```python
from build123d import *

# Parameters (mm, degrees)
EXTRUDE_1_DEPTH     = 2
SKETCH_2_W          = 90
SKETCH_2_H          = 11
CUT_EXTRUDE_1_DEPTH = 2
SKETCH_4_W          = 10
SKETCH_4_H          = 11
SKETCH_4_R          = 1.65
EXTRUDE_3_DEPTH     = 2
FILLET_2_R          = 2


with BuildPart() as part:
    # 草图1 → 凸台-拉伸1 (new body)
    with BuildSketch(Plane.XY):
        Polygon((-33, -15), (-52.5, -15), (-52.5, 15), (-33, 15), (-33, 17), (-23, 17), (-23, 15), (23, 15), (23, 17), (33, 17), (33, 15), (52.5, 15), (52.5, -15), (33, -15), (33, -17), (23, -17), (23, -15), (-23, -15), (-23, -17), (-33, -17), align=None)
    extrude(amount=EXTRUDE_1_DEPTH)

    # 草图2 → 切除-拉伸1 (cut)
    with BuildSketch(Plane.XY.offset(2)):
        Rectangle(SKETCH_2_W, SKETCH_2_H)
    extrude(amount=-CUT_EXTRUDE_1_DEPTH, mode=Mode.SUBTRACT)

    # 草图4 → 凸台-拉伸3 (add)
    # profile 1 of 2: a face of its own
    with BuildSketch(Plane(origin=(0, 0, 0), x_dir=(-1, 0, 0), z_dir=(0, 0, -1))):
        with Locations((-22.5, 0)):
            Rectangle(SKETCH_4_W, SKETCH_4_H)
        with Locations((-22.5, 0)):
            Circle(SKETCH_4_R, mode=Mode.SUBTRACT)
    # profile 2 of 2: a face of its own
    with BuildSketch(Plane(origin=(0, 0, 0), x_dir=(-1, 0, 0), z_dir=(0, 0, -1))):
        with Locations((22.5, 0)):
            Rectangle(SKETCH_4_W, SKETCH_4_H)
        with Locations((22.5, 0)):
            Circle(SKETCH_4_R, mode=Mode.SUBTRACT)
    extrude(amount=-EXTRUDE_3_DEPTH)

    # 圆角2
    fillet_2_edges = [part.edges().sort_by_distance(p)[0] for p in [
        (-45, -5.5, 1),
        (-45, 5.5, 1),
        (45, 5.5, 1),
        (45, -5.5, 1),
        (17.5, -5.5, 1),
        (17.5, 5.5, 1),
        (27.5, 5.5, 1),
        (27.5, -5.5, 1),
        (-27.5, -5.5, 1),
        (-27.5, 5.5, 1),
        (-17.5, 5.5, 1),
        (-17.5, -5.5, 1),
    ]]
    fillet(fillet_2_edges, radius=FILLET_2_R)


solid = part.part
```
Input: part model. Units: mm. Frame: model coordinates. A direction names the side the tool comes from. Coordinates: 2 decimals unless noted, no trailing zeros. Loops run counter-clockwise (first coordinate to the right, second up) from the corner with the lowest first, then second, coordinate; pieces in that order, holes last. Notation, with made-up numbers: M 12,49 L 17,49 A23 ccw 17,62 Z; hole C -11.5,72 d1. An arc over 180 degrees is marked long. One line per item, written item: value.
(1) Section C-C (z = 0.7). Give the number of separate pieces and of enclosed holes in the cut face, and give its area (3 significant figures).
Filled in:
separate pieces: 1
enclosed holes: 5
area: 2,450 mm^2
(2) Line query: line 1 along Y through (x, z) = (22.5, 0.95); line 2 along Y through (x, z) = (-32, 0.35); line 3 along X through (y, z) = (-2.5, 0.85). Output: solid intervals per line, ascending. Write a range as from..to.
Filled in:
line 1: -15..-1.65, 1.65..15
line 2: -17..-5.5, 5.5..17
line 3: -52.5..-45, -27.5..-17.5, 17.5..27.5, 45..52.5
(3) Section A-A (y = 0). Output: boundary loops of the cut face in (x, z).
Filled in:
outline: M -52.5,0 L -45,0 L -45,2 L -52.5,2 Z; M -27.5,0 L -24.15,0 L -24.15,2 L -27.5,2 Z; M -20.85,0 L -17.5,0 L -17.5,2 L -20.85,2 Z; M 17.5,0 L 20.85,0 L 20.85,2 L 17.5,2 Z; M 24.15,0 L 27.5,0 L 27.5,2 L 24.15,2 Z; M 45,0 L 52.5,0 L 52.5,2 L 45,2 Z
(4) Pin query (flat end, axial travel): pin 1 (1 mm diameter, centred on x = -9, z = 0.5, fed in from -Y); pin 2 (1 mm diameter, centred on y = 16, z = 1.5, fed in from -X); pin 3 (0.6 mm diameter, centred on x = 8, z = 0.5, fed in from +Y). Return the tip coordinate at first contact, or that it passes through.
Filled in:
pin 1: y = -15
pin 2: x = -33
pin 3: y = 15
(5) Reachability of faces 4 (the flat face through (33, -16, 1)), 5 (the cylindrical face through (-16.9, 4.93, 1.01)), 6 (the flat face through (-33, 16, 1)), 7 (the flat face through (43, 15, 1)) from +Z, -Z, +X, -X, +Y, -Y: full face, straight path, thin tool, end or side. Return the list, or none.
Filled in:
face 4: +Z, -Z, +X, -Y
face 5: +Z, -Z
face 6: +Z, -Z, -X, +Y
face 7: +Z, -Z, +X, +Y
(6) Section B-B (x = 35.5). Output: boundary loops of the cut face in (y, z).
Filled in:
outline: M -15,0 L -5.5,0 L -5.5,2 L -15,2 Z; M 5.5,0 L 15,0 L 15,2 L 5.5,2 Z
(7) Pull-direction query (Y, two-part tool) for faces 1 (the flat face through (-17.5, 0, 1)), 2 (the flat face through (23, -16, 1)), 3 (the flat face through (0, 15, 1)); classes: +Y half, -Y half, draft (parallel to the pull), parting line (faces both ways), or undercut.
Filled in:
face 1: undercut
face 2: draft
face 3: +Y half
